Model file for the job. Use its own axes, mm. A direction names the side the tool comes from. Round coordinates to 2 decimals unless told otherwise and drop trailing zeros. Order: outer loops, then holes, each group sorted by start corner. A loop starts at its lowest first (then second) coordinate and runs counter-clockwise, first axis right, second up. Notation, with made-up numbers: (64.5, 3.25) - (83.5, 3.25) arc R16 ccw to (83.5, 9.25) - close; hole circle Ø4 at (-14.5, 64.25). An arc over 180 degrees is marked (long way). Put each result on its own line as item: value. Start each with the question number.
Item 1: Saw through at D-D on y = 55. List the corners of the cut face in (x, z) (3 decimals).
Item 2: Saw through at B-B on z = 0.85. State how many separate pieces and enclosed holes the cut face has, plus the area to 3 significant figures.
Item 3: Which spindle directions (+Z, -Z, +X, -X, +Y, -Y) get a long thin tool onto all of the face, cutting with end or side? Do faces 1 (the face through (7.888, 103.847, 1.565)), 2 (the face through (61, 10, 3.175)). Say none if no direction does.
Item 4: Saw through at A-A on y = 6.35. List the corners of the cut face in (x, z) (1 decimal), plus the area to 3 significant figures.
Item 5: Saw through at C-C on x = 66.5. List the corners of the cut face in (y, z) (3 decimals), plus the area to 3 significant figures.
Item 6: Probe probe 1 along X at (y, z) = (41.5, 1.65) (3 decimals); probe 2 along Y at (x, z) = (86, 0.9); probe 3 along Y at (x, z) = (136.5, 0.15). List the from-to ranges inside material, lowest first.
Item 7: Mould opens along Y. For faces 3 (the face through (70, 0, 2)), 4 (the face through (132.78, 6.44, 1.57)), 5 (the face through (61, 10, 0)) say: pulls with the +Y half, pulls with the -Y half, needs draft (parallel to the pull), parting line crosses it, or undercut.
```python
from build123d import *

# Parameters (mm, degrees)
SKETCH1_R           = 2.159
SKETCH1_W           = 111.125
SKETCH1_H           = 82.55
BOSS_EXTRUDE1_DEPTH = 3.175


with BuildPart() as part:
    # Sketch1 → Boss-Extrude1 (new body)
    with BuildSketch(Plane.XY):
        Polygon((0, 0), (15.875, 0), (127, 0), (142.875, 0), (142.875, 107.95), (127, 107.95), (15.875, 107.95), (0, 107.95), align=None)
        with Locations((7.9375, 6.35)):
            Circle(SKETCH1_R, mode=Mode.SUBTRACT)
        with Locations((134.9375, 6.35)):
            Circle(SKETCH1_R, mode=Mode.SUBTRACT)
        with BuildLine():
            Line((10.1854, 101.6), (10.1854, 21.59))
            ThreePointArc((10.1854, 21.59), (7.9375, 19.3421), (5.6896, 21.59))
            Line((5.6896, 21.59), (5.6896, 101.6))
            ThreePointArc((5.6896, 101.6), (7.9375, 103.8479), (10.1854, 101.6))
        make_face(mode=Mode.SUBTRACT)
        with Locations((71.4375, 53.975)):
            Rectangle(SKETCH1_W, SKETCH1_H, mode=Mode.SUBTRACT)
        with BuildLine():
            Line((132.6896, 101.6), (132.6896, 21.59))
            ThreePointArc((132.6896, 21.59), (134.9375, 19.3421), (137.1854, 21.59))
            Line((137.1854, 21.59), (137.1854, 101.6))
            ThreePointArc((137.1854, 101.6), (134.9375, 103.8479), (132.6896, 101.6))
        make_face(mode=Mode.SUBTRACT)
    extrude(amount=BOSS_EXTRUDE1_DEPTH)


solid = part.part
```
Results found:
1. outline: (0, 0) - (5.69, 0) - (5.69, 3.175) - (0, 3.175) - close; (10.185, 0) - (15.875, 0) - (15.875, 3.175) - (10.185, 3.175) - close; (127, 0) - (132.69, 0) - (132.69, 3.175) - (127, 3.175) - close; (137.185, 0) - (142.875, 0) - (142.875, 3.175) - (137.185, 3.175) - close
2. separate pieces: 1
2. enclosed holes: 5
2. area: 5,470 mm²
3. face 1: +Z, -Z
3. face 2: +Z, +X, -X, +Y, -Y
4. outline: (0, 0) - (5.8, 0) - (5.8, 3.2) - (0, 3.2) - close; (10.1, 0) - (132.8, 0) - (132.8, 3.2) - (10.1, 3.2) - close; (137.1, 0) - (142.9, 0) - (142.9, 3.2) - (137.1, 3.2) - close
4. area: 426 mm²
5. outline: (0, 0) - (12.7, 0) - (12.7, 3.175) - (0, 3.175) - close; (95.25, 0) - (107.95, 0) - (107.95, 3.175) - (95.25, 3.175) - close
5. area: 80.6 mm²
6. probe 1: x = 0 to 5.69, 10.185 to 15.875, 127 to 132.69, 137.185 to 142.875
6. probe 2: y = 0 to 12.7, 95.25 to 107.95
6. probe 3: y = 0 to 4.86, 7.84 to 19.97, 103.22 to 107.95
7. face 3: pulls with the -Y half
7. face 4: undercut
7. face 5: needs draft
